Work out the finished part from the listing and answer in its coordinate system (mm). Give positions to 0.01 mm unless a question says otherwise; leave off trailing zeros. Loops run counter-clockwise (first coordinate to the right, second up) from the corner with the lowest first, then second, coordinate; pieces in that order, holes last. Notation, with made-up numbers: (13.25, 19.5) - (43.25, 19.5) arc R4 cw to (43.25, 25.5) - close; hole circle Ø7 at (-22.75, 53.5). An arc over 180 degrees is marked (long way). One line per question, with ' | ' between items. Start each with the question number.
1. Section D-D (y = -8) is taken. Determine the outline of the cut face in (x, z).
2. Section B-B (x = 107.5) is taken. Determine the outline of the cut face in (y, z).
3. Section C-C (z = 3.9) is taken. Give the number of separate pieces and of enclosed holes in the cut face, plus the area to 3 significant figures.
4. Section A-A (y = 0) is taken. Determine the outline of the cut face in (x, z).
5. Find the intervals of material crossed by line 1 (Y direction, x = 23.5, z = 4.35); line 2 (X direction, y = 5.5, z = 3.7); line 3 (X direction, y = 6, z = 4.85), in increasing order.
6. This flat-tipped pin is pushed along its axis until it touches: pin 1 (2.5 mm diameter, centred on y = 1.5, z = 3.5, fed in from -X). Where does it stop, or does it pass through?
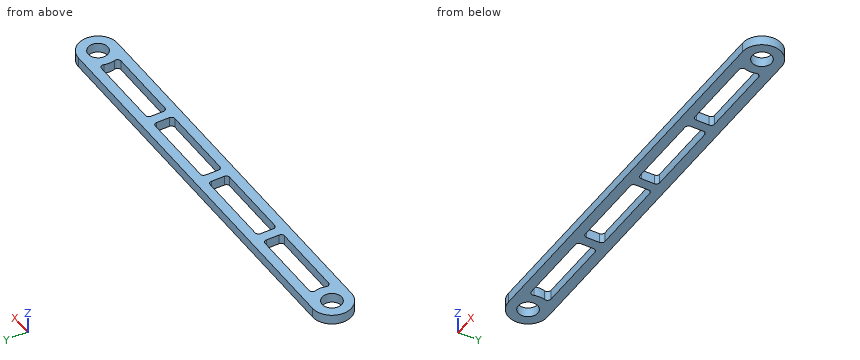
from build123d import *

# Parameters (mm, degrees)
SKETCH_1_R      = 5
EXTRUDE_1_DEPTH = 5


with BuildPart() as part:
    # 草图1 → 凸台-拉伸1 (new body)
    with BuildSketch(Plane.XY):
        with BuildLine():
            Line((0, 10), (200, 10))
            ThreePointArc((200, 10), (210, 0), (200, -10))
            Line((200, -10), (0, -10))
            ThreePointArc((0, -10), (-10, 0), (0, 10))
        make_face()
        Circle(SKETCH_1_R, mode=Mode.SUBTRACT)
        with Locations((200, 0)):
            Circle(SKETCH_1_R, mode=Mode.SUBTRACT)
        with BuildLine():
            Line((11.245449786, 5), (48.864788989, 5))
            ThreePointArc((48.864788989, 5), (50.077716142, 4.497589123), (50.580127019, 3.28466197))
            Line((50.580127019, 3.28466197), (50.580127019, 0))
            Line((50.580127019, 0), (50.580127019, -3.28466197))
            ThreePointArc((50.580127019, -3.28466197), (50.077716142, -4.497589123), (48.864788989, -5))
            Line((48.864788989, -5), (11.245449786, -5))
            ThreePointArc((11.245449786, -5), (9.872979547, -4.313598314), (9.59891192, -2.803727867))
            ThreePointArc((9.59891192, -2.803727867), (10, 0), (9.59891192, 2.803727867))
            ThreePointArc((9.59891192, 2.803727867), (9.872979547, 4.313598314), (11.245449786, 5))
        make_face(mode=Mode.SUBTRACT)
        with BuildLine():
            Line((188.754550214, -5), (151.135211011, -5))
            ThreePointArc((151.135211011, -5), (149.922283858, -4.497589123), (149.419872981, -3.28466197))
            Line((149.419872981, -3.28466197), (149.419872981, 0))
            Line((149.419872981, 0), (149.419872981, 3.28466197))
            ThreePointArc((149.419872981, 3.28466197), (149.922283858, 4.497589123), (151.135211011, 5))
            Line((151.135211011, 5), (188.754550214, 5))
            ThreePointArc((188.754550214, 5), (190.127020453, 4.313598314), (190.40108808, 2.803727867))
            ThreePointArc((190.40108808, 2.803727867), (190, 0), (190.40108808, -2.803727867))
            ThreePointArc((190.40108808, -2.803727867), (190.127020453, -4.313598314), (188.754550214, -5))
        make_face(mode=Mode.SUBTRACT)
        with BuildLine():
            Line((104.21533803, 5), (142.704534951, 5))
            ThreePointArc((142.704534951, 5), (143.917462104, 4.497589123), (144.419872981, 3.28466197))
            Line((144.419872981, 3.28466197), (144.419872981, 0))
            Line((144.419872981, 0), (144.419872981, -3.28466197))
            ThreePointArc((144.419872981, -3.28466197), (143.917462104, -4.497589123), (142.704534951, -5))
            Line((142.704534951, -5), (104.21533803, -5))
            ThreePointArc((104.21533803, -5), (103.002410877, -4.497589123), (102.5, -3.28466197))
            Line((102.5, -3.28466197), (102.5, 0))
            Line((102.5, 0), (102.5, 3.28466197))
            ThreePointArc((102.5, 3.28466197), (103.002410877, 4.497589123), (104.21533803, 5))
        make_face(mode=Mode.SUBTRACT)
        with BuildLine():
            Line((95.78466197, -5), (57.295465049, -5))
            ThreePointArc((57.295465049, -5), (56.082537896, -4.497589123), (55.580127019, -3.28466197))
            Line((55.580127019, -3.28466197), (55.580127019, 0))
            Line((55.580127019, 0), (55.580127019, 3.28466197))
            ThreePointArc((55.580127019, 3.28466197), (56.082537896, 4.497589123), (57.295465049, 5))
            Line((57.295465049, 5), (95.78466197, 5))
            ThreePointArc((95.78466197, 5), (96.997589123, 4.497589123), (97.5, 3.28466197))
            Line((97.5, 3.28466197), (97.5, 0))
            Line((97.5, 0), (97.5, -3.28466197))
            ThreePointArc((97.5, -3.28466197), (96.997589123, -4.497589123), (95.78466197, -5))
        make_face(mode=Mode.SUBTRACT)
    extrude(amount=EXTRUDE_1_DEPTH)


solid = part.part
Conclusion:
1) outline: (-6, 0) - (206, 0) - (206, 5) - (-6, 5) - close
2) outline: (-10, 0) - (-5, 0) - (-5, 5) - (-10, 5) - close; (5, 0) - (10, 0) - (10, 5) - (5, 5) - close
3) separate pieces: 1 | enclosed holes: 6 | area: 2,510 mm²
4) outline: (-10, 0) - (-5, 0) - (-5, 5) - (-10, 5) - close; (5, 0) - (10, 0) - (10, 5) - (5, 5) - close; (50.58, 0) - (55.58, 0) - (55.58, 5) - (50.58, 5) - close; (97.5, 0) - (102.5, 0) - (102.5, 5) - (97.5, 5) - close; (144.42, 0) - (149.42, 0) - (149.42, 5) - (144.42, 5) - close; (190, 0) - (195, 0) - (195, 5) - (190, 5) - close; (205, 0) - (210, 0) - (210, 5) - (205, 5) - close
5) line 1: -10 to -5, 5 to 10 | line 2: -8.35 to 208.35 | line 3: -8 to 208
6) pin 1: x = -10
